Source: CAD feature listing. Evaluate the final solid. Frame: model axes, mm. Face numbers are marked on the shaded views. Round coordinates to 2 decimals unless told otherwise and drop trailing zeros. Write each loop counter-clockwise with the first axis right and the second up, starting at its lowest first coordinate (ties: lowest second). Pieces come first, ordered by that corner, then holes.
from build123d import *

# Parameters (mm, degrees)
F0_R     = 31.75
F0_R_2   = 27.94
F1_DEPTH = 76.2
F4_R     = 0.254


with BuildPart() as f1:
    # F0 (on Front) → F1 (new body, symmetric)
    with BuildSketch(Plane.XZ):
        Circle(F0_R)
        Circle(F0_R_2, mode=Mode.SUBTRACT)
    extrude(amount=F1_DEPTH, both=True)

    # F2 (on Top) → F3 (revolve)
    with BuildSketch(Plane.XY):
        Polygon((31.75, -76.2), (27.94, -76.2), (2.54, -116.84), (2.54, -122.936), align=None)
    revolve(axis=Axis((0, -64.747475, 0), (0, -1, 0)))

    # F4
    f4_edges = [f1.edges().sort_by_distance(p)[0] for p in [
        (-2.54, -122.936, 0),
    ]]
    fillet(f4_edges, radius=F4_R)


solid = f1.part
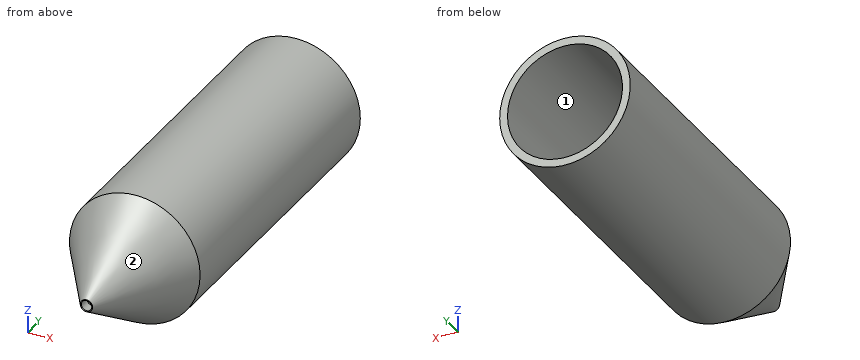
1) Section query A-A on y = -89. Return the cut outline in (x, z).
Taken from the geometry:
outline: circle Ø47.5 at (0, 0); hole circle Ø39.88 at (0, 0)
2) Material intervals for line 1 (Z direction, x = 0, y = -2); line 2 (Z direction, x = -9.5, y = -103); line 3 (X direction, y = 29, z = -22), sorted ascending.
Taken from the geometry:
line 1: z = -31.75 to -27.94, 27.94 to 31.75
line 2: z = -11.61 to -5.91, 5.91 to 11.61
line 3: x = -22.89 to -17.22, 17.22 to 22.89
3) Section query B-B on y = -53.5. Return the cut outline in (x, z), then the cut area to 3 significant figures.
Taken from the geometry:
outline: circle Ø63.5 at (0, 0); hole circle Ø55.88 at (0, 0)
area: 714 mm2
4) Contact query for flat-ended pins moving along their axis: P1, Ø8, axis at x = 10, y = 46, coming from the +Z side; P2, Ø1, axis at x = -7, y = -77, coming from the -Z side; P3, Ø1.5, axis at x = -22.5, y = 46, coming from the +Z side; P4, Ø6, axis at x = 0, z = 0, coming from the -Y side. Output: stop coordinate, or through.
Taken from the geometry:
P1: stops at z = 31.18
P2: stops at z = -30.8
P3: stops at z = 23.13
P4: stops at y = -122.3
5) Pull-direction query (Z, two-part tool) for the marked faces 1 and 2; classes: released by +Z, released by -Z, zero draft, split by the parting line, or undercut.
Taken from the geometry:
face 1: undercut
face 2: split by the parting line
